```python
from build123d import *

# Parameters (mm, degrees)
SKETCH2_W          = 25.4
SKETCH2_H          = 10.16
SKETCH3_W          = 6.35
SKETCH3_H          = 38.1
CUT_EXTRUDE1_DEPTH = 1.27


with BuildPart() as part:
    # Sketch2 → Revolve1 (revolve)
    with BuildSketch(Plane(origin=(0, 0, 0), x_dir=(1, 0, 0), z_dir=(0, 1, 0)), mode=Mode.PRIVATE) as revolve1_sk:
        with Locations((12.7, 0)):
            Rectangle(SKETCH2_W, SKETCH2_H)
        Polygon((25.4, 5.08), (25.4, -5.08), (25.4, -6.35), (31.75, -6.35), (31.75, 6.35), (25.4, 6.35), align=None)
    revolve(revolve1_sk.sketch.rotate(Axis((0, 0, -88.99), (0, 0, 1)), 180), axis=Axis((0, 0, -88.99), (0, 0, 1)))

    # Sketch3 → Cut-Extrude1 (cut)
    with BuildSketch(Plane.XY.offset(5.08)):
        Rectangle(SKETCH3_W, SKETCH3_H)
    cut_extrude1 = extrude(amount=-CUT_EXTRUDE1_DEPTH, mode=Mode.SUBTRACT)

    # Mirror1: Cut-Extrude1 across plane
    add(cut_extrude1.mirror(Plane.XY), mode=Mode.SUBTRACT)


solid = part.part
```
Can you work these out from the model? Positions are in its coordinate system, mm. A direction names the side the tool comes from. Round coordinates to 2 decimals unless told otherwise and drop trailing zeros. Order: outer loops, then holes, each group sorted by start corner. A loop starts at its lowest first (then second) coordinate and runs counter-clockwise, first axis right, second up.
(1) If we section it at D-D (x = 20): Please give me the cut outline in (y, z).
Results are:
outline: (-24.66, -6.35) - (-15.66, -6.35) - (-15.66, -5.08) - (15.66, -5.08) - (15.66, -6.35) - (24.66, -6.35) - (24.66, 6.35) - (15.66, 6.35) - (15.66, 5.08) - (-15.66, 5.08) - (-15.66, 6.35) - (-24.66, 6.35) - close
(2) If we section it at C-C (z = 0.5): Please give me the cut outline in (x, y), plus the area to 3 significant figures.
Results are:
outline: circle Ø63.5 at (0, 0)
area: 3,170 mm2
(3) We'd pull the mould along Y, two halves only. Please class faces 4 (the face through (6.883, 30.995, -0.089)), 5 (the face through (14.3, -21.3, -6.35)), 6 (the face through (0, 0, 3.81)): +Y half, -Y half, draft (parallel to the pull), parting line (faces both ways), or undercut.
Results are:
face 4: parting line
face 5: draft
face 6: undercut
(4) If we section it at B-B (y = 0): Please give me the cut outline in (x, z) (3 decimals).
Results are:
outline: (-31.75, -6.35) - (-25.4, -6.35) - (-25.4, -5.08) - (-3.175, -5.08) - (-3.175, -3.81) - (3.175, -3.81) - (3.175, -5.08) - (25.4, -5.08) - (25.4, -6.35) - (31.75, -6.35) - (31.75, 6.35) - (25.4, 6.35) - (25.4, 5.08) - (3.175, 5.08) - (3.175, 3.81) - (-3.175, 3.81) - (-3.175, 5.08) - (-25.4, 5.08) - (-25.4, 6.35) - (-31.75, 6.35) - close
(5) If I drill on L1, parallel to Y at x = 0, z = -5.8; L2, parallel to Z at x = -9, y = 17; L3, parallel to Y at x = -17.5, z = -5.5, over which ranges is the centre line in solid material (lowest first)?
Results are:
L1: y = -31.75 to -25.4, 25.4 to 31.75
L2: z = -5.08 to 5.08
L3: y = -26.49 to -18.41, 18.41 to 26.49
(6) I'm going to push flat-ended pins straight in: pin 1 (5 mm diameter, centred on x = 0.5, y = 6.5, fed in from -Z); pin 2 (5 mm diameter, centred on x = 22, z = -2.5, fed in from +Y); pin 3 (0.6 mm diameter, centred on y = -6, z = 4.5, fed in from +X). Where does each tip first touch, or does it pass through?
Results are:
pin 1: stops at z = -3.81
pin 2: stops at y = 25.06
pin 3: stops at x = 31.23
(7) If we section it at A-A (x = 0): Please give me the cut outline in (y, z), plus the area to 3 significant figures.
Results are:
outline: (-31.75, -6.35) - (-25.4, -6.35) - (-25.4, -5.08) - (-19.05, -5.08) - (-19.05, -3.81) - (19.05, -3.81) - (19.05, -5.08) - (25.4, -5.08) - (25.4, -6.35) - (31.75, -6.35) - (31.75, 6.35) - (25.4, 6.35) - (25.4, 5.08) - (19.05, 5.08) - (19.05, 3.81) - (-19.05, 3.81) - (-19.05, 5.08) - (-25.4, 5.08) - (-25.4, 6.35) - (-31.75, 6.35) - close
area: 581 mm2
(8) On a 3-axis mill with a long thin cutter (end or side, diameter ignored), from which of +Z, -Z, +X, -X, +Y, -Y can I reach the whole of each face in a straight line? I mean faces 1 (the face through (-14.3, -21.3, 6.35)), 2 (the face through (5, 0, 5.08)), 3 (the face through (-11.721, 22.534, -5.706)). Say none if no direction works.
Results are:
face 1: +Z, +X, -X, +Y, -Y
face 2: +Z
face 3: -Z
